Input: dimensioned drawing with shaded views. Units: mm. Origin: part minimum x, y, z. Give positions to 0.01 mm unless a question says otherwise; leave off trailing zeros. Write each loop counter-clockwise with the first axis right and the second up, starting at its lowest first coordinate (ties: lowest second). Pieces come first, ordered by that corner, then holes.
Q1. Section D-D (x = 103). Return the cut outline in (y, z), plus the area to 3 significant figures.
Q2. Section A-A (z = 74.5). Return the cut outline in (x, y), plus the area to 3 significant figures.
Q3. Pin query (flat end, axial travel): pin 1 Ø6 at (x, y) = (91, 4.5) entering from -Z; pin 2 Ø5 at (x, z) = (89.5, 34.5) entering from +Y; pin 3 Ø5 at (x, y) = (119, 7) entering from +Z. Return the tip coordinate at first contact, or that it passes through.
Q4. Line query: line 1 (Z direction, x = 74.5, y = 8.15); line 2 (X direction, y = 4.25, z = 63.5); line 3 (X direction, y = 2.25, z = 74.5). Output: solid intervals per line, ascending.
Q5. Section B-B (x = 74.5). Return the cut outline in (y, z), plus the area to 3 significant figures.
Q6. Section C-C (y = 6.25). Return the cut outline in (x, z).
Q7. Mould query, pull axis Z, two halves, no side actions, for the marked faces 1 and 2. Classes: +Z half, -Z half, draft (parallel to the pull), parting line (faces both ways), or undercut.
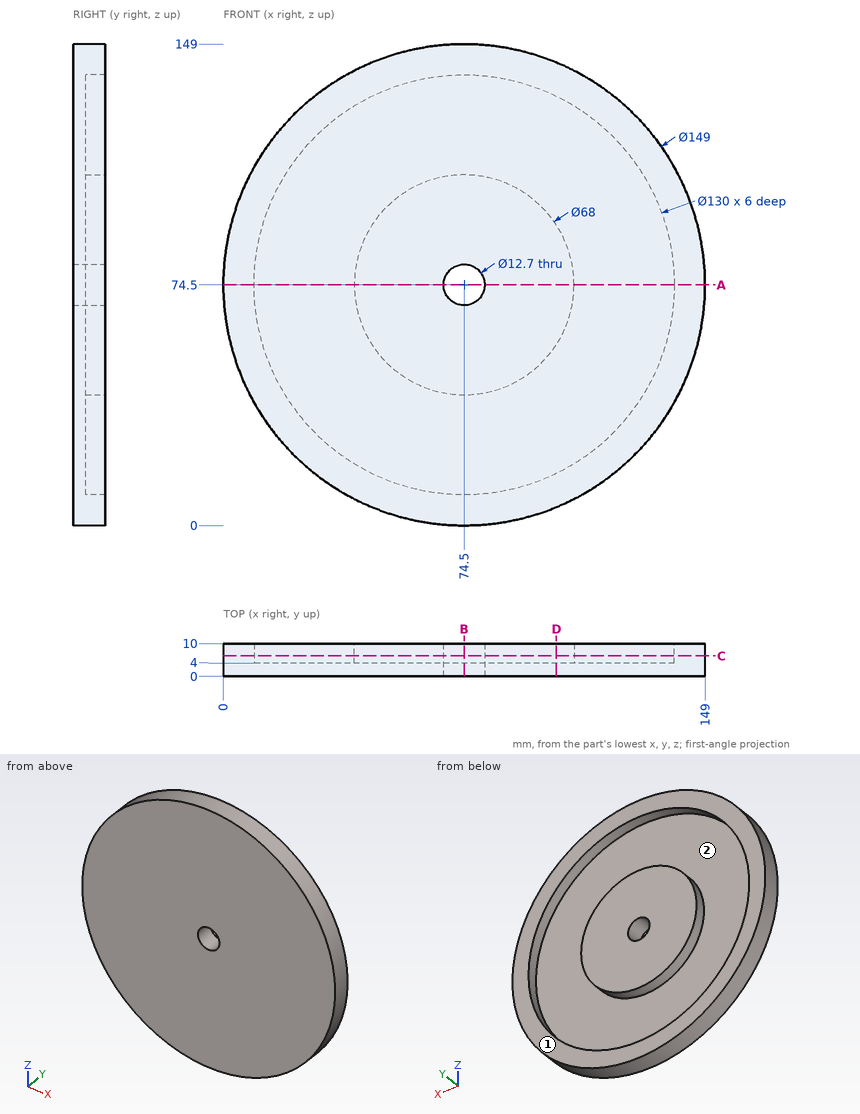
Computed:
1. outline: (0, 5.67) - (10, 5.67) - (10, 16.08) - (4, 16.08) - (4, 55.96) - (10, 55.96) - (10, 93.04) - (4, 93.04) - (4, 132.92) - (10, 132.92) - (10, 143.33) - (0, 143.33) - close
1. area: 898 mm2
2. outline: (0, 0) - (68.15, 0) - (68.15, 10) - (40.5, 10) - (40.5, 4) - (9.5, 4) - (9.5, 10) - (0, 10) - close; (80.85, 0) - (149, 0) - (149, 10) - (139.5, 10) - (139.5, 4) - (108.5, 4) - (108.5, 10) - (80.85, 10) - close
2. area: 991 mm2
3. pin 1: stops at z = 1.23
3. pin 2: stops at y = 4
3. pin 3: stops at z = 136.03
4. line 1: z = 0 to 9.5, 40.5 to 68.15, 80.85 to 108.5, 139.5 to 149
4. line 2: x = 0.82 to 10.44, 42.33 to 106.67, 138.56 to 148.18
4. line 3: x = 0 to 68.15, 80.85 to 149
5. outline: (0, 0) - (10, 0) - (10, 9.5) - (4, 9.5) - (4, 40.5) - (10, 40.5) - (10, 68.15) - (0, 68.15) - close; (0, 80.85) - (10, 80.85) - (10, 108.5) - (4, 108.5) - (4, 139.5) - (10, 139.5) - (10, 149) - (0, 149) - close
5. area: 991 mm2
6. outline: circle Ø149 at (74.5, 74.5); circle Ø68 at (74.5, 74.5); hole circle Ø130 at (74.5, 74.5); hole circle Ø12.7 at (74.5, 74.5)
7. face 1: draft
7. face 2: undercut
